Design review of the part built by this model. Coordinates are the model's own, in mm. Face numbers are marked on the shaded views. Coordinates: 2 decimals unless noted, no trailing zeros. Loops run counter-clockwise (first coordinate to the right, second up) from the corner with the lowest first, then second, coordinate; pieces in that order, holes last. Notation, with made-up numbers: (34.25, 64) - (70.25, 64) arc R29 ccw to (70.25, 92) - close; hole circle Ø2 at (-13.75, 45.5). An arc over 180 degrees is marked (long way). Answer in a Markdown table with one row per item. Add a question column.
(1) We need section C-C, the plane z = 19.75. Write out the cut boundary in (x, y).
(2) We need section A-A, the plane y = 0. Write out the cut boundary in (x, z).
(3) We need section D-D, the plane x = -8. Write out the cut boundary in (y, z), plus the area to 3 significant figures.
(4) The part is to be moulded in two halves that separate along Y. For the marked faces 1, 2 and 3, say which applies: released by +Y, released by -Y, zero draft, split by the parting line, or undercut.
(5) Clearance check with flat-ended pins moving along their axes: pin 1 (2 mm diameter, centred on y = -16, z = 3, fed in from +X); pin 2 (1.8 mm diameter, centred on x = 0, y = 0, fed in from -Z); pin 3 (1.5 mm diameter, centred on y = 8.5, z = 8, fed in from -X); pin 4 (12 mm diameter, centred on x = 6, z = 13, fed in from -Y). State where each tip first meets the part, or that it passes through.
(6) To check wall thickness, follow L1, parallel to Y at x = 0, z = 14; L2, parallel to Y at x = 0, z = 25.65; L3, parallel to X at y = 11, z = 5. State the ranges of each line that lie inside material, in increasing order. Write a range as [from, to].
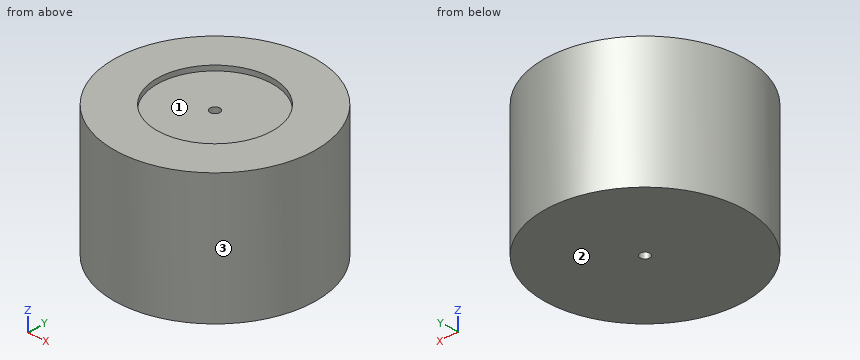
from build123d import *

# Parameters (mm, degrees)
F0_R     = 20
F1_DEPTH = 25
F2_D     = 2
F2_DEPTH = 27
F2_TIP   = 0.600860619
F3_R     = 20
F4_DEPTH = 1
F5_D     = 23
F5_DEPTH = 4
F5_TIP   = 6.9098971188


with BuildPart() as f1:
    # F0 (on Top) → F1 (new body)
    with BuildSketch(Plane.XY):
        Circle(F0_R)
    extrude(amount=F1_DEPTH)

    # F2
    with Locations(Plane(origin=(0, 0, 0), x_dir=(1, 0, 0), z_dir=(0, 0, -1))):
        with Locations((0, 0)):
            Hole(F2_D / 2, depth=F2_DEPTH)
            with Locations((0, 0, -(F2_DEPTH + F2_TIP / 2))):  # 118° drill point
                Cone(0, F2_D / 2, F2_TIP, mode=Mode.SUBTRACT)

    # F3 (on face) → F4 (join)
    with BuildSketch(Plane.XY.offset(25)):
        Circle(F3_R)
    extrude(amount=F4_DEPTH)

    # F5 (one way)
    with BuildSketch(Plane(origin=(0, 0, 25), x_dir=(1, 0, 0), z_dir=(0, 0, -1))):
        with Locations((0, 0)):
            Circle(F5_D / 2)
    extrude(amount=-F5_DEPTH, mode=Mode.SUBTRACT)
    with Locations(Plane(origin=(0, 0, 25), x_dir=(1, 0, 0), z_dir=(0, 0, -1))):
        with Locations((0, 0)):
            with Locations((0, 0, -(F5_DEPTH + F5_TIP / 2))):  # 118° drill point
                Cone(0, F5_D / 2, F5_TIP, mode=Mode.SUBTRACT)


solid = f1.part
Responses:
| question | item | result |
|---|---|---|
| 1 | outline | circle Ø40 at (0, 0); hole circle Ø2 at (0, 0) |
| 2 | outline | (-20, 0) - (-1, 0) - (-1, 25) - (-11.5, 25) - (-11.5, 26) - (-20, 26) - close; (1, 0) - (20, 0) - (20, 26) - (11.5, 26) - (11.5, 25) - (1, 25) - close |
| 3 | outline | (-18.33, 0) - (18.33, 0) - (18.33, 26) - (8.26, 26) - (8.26, 25) - (-8.26, 25) - (-8.26, 26) - (-18.33, 26) - close |
| 3 | area | 937 mm2 |
| 4 | face 1 | undercut |
| 4 | face 2 | zero draft |
| 4 | face 3 | split by the parting line |
| 5 | pin 1 | stops at x = 13.23 |
| 5 | pin 2 | passes through |
| 5 | pin 3 | stops at x = -18.44 |
| 5 | pin 4 | stops at y = -20 |
| 6 | L1 | y = [-20, -1], [1, 20] |
| 6 | L2 | y = [-20, -11.5], [11.5, 20] |
| 6 | L3 | x = [-16.7, 16.7] |
